```python
from build123d import *

# Parameters (mm, degrees)
CROQUIS3_R              = 2.5103265
CROQUIS3_R_2            = 2.5
SALIENTE_EXTRUIR1_DEPTH = 4


with BuildPart() as part:
    # Croquis3 → Saliente-Extruir1 (new body)
    with BuildSketch(Plane(origin=(0, 0, 0), x_dir=(0, 0, -1), z_dir=(1, 0, 0))):
        with BuildLine():
            Line((5, 0), (5, -25))
            Line((5, -25), (-20, -25))
            ThreePointArc((-20, -25), (-24.631788644, -18.116775648), (-16.510921132, -16.418613585))
            ThreePointArc((-16.510921132, -16.418613585), (-9.814593541, -8.868938988), (-5, 0))
            ThreePointArc((-5, 0), (0, 5), (5, 0))
        make_face()
        Circle(CROQUIS3_R, mode=Mode.SUBTRACT)
        with Locations((-20, -20)):
            Circle(CROQUIS3_R_2, mode=Mode.SUBTRACT)
    extrude(amount=SALIENTE_EXTRUIR1_DEPTH)


solid = part.part
```
The listing builds one solid part. Answer for the finished solid, in the listing's coordinates (mm). Round coordinates to 2 decimals unless told otherwise and drop trailing zeros. Loops run counter-clockwise (first coordinate to the right, second up) from the corner with the lowest first, then second, coordinate; pieces in that order, holes last.
1) A cutting plane is placed at D-D on z = 23. Determine the outline of the cut face in (x, y).
Outcome:
outline: (0, -24) - (4, -24) - (4, -16) - (0, -16) - close
2) For a pull along Z with two mould halves and no side action, classify faces 1 (the face through (2, -12, -5)), 2 (the face through (4, -13, 6)), 3 (the face through (2, -19.9, 22.5)) as released by +Z, released by -Z, zero draft, split by the parting line, or undercut.
Outcome:
face 1: released by -Z
face 2: zero draft
face 3: undercut
3) A cutting plane is placed at B-B on z = 0. Determine the outline of the cut face in (x, y), plus the area to 3 significant figures.
Outcome:
outline: (0, -25) - (4, -25) - (4, -2.51) - (0, -2.51) - close; (0, 2.51) - (4, 2.51) - (4, 5) - (0, 5) - close
area: 99.9 mm2
4) Consider line 1 (Y direction, x = 2.1, z = 0); line 2 (Y direction, x = 1.4, z = 20); line 3 (Z direction, x = 0.2, y = -1.5). Determine where each line is inside the solid, lowest interval first.
Outcome:
line 1: y = -25 to -2.51, 2.51 to 5
line 2: y = -25 to -22.5, -17.5 to -15
line 3: z = -5 to -2.01, 2.01 to 5.64
5) A cutting plane is placed at A-A on y = -20. Determine the outline of the cut face in (x, z).
Outcome:
outline: (0, -5) - (4, -5) - (4, 17.5) - (0, 17.5) - close; (0, 22.5) - (4, 22.5) - (4, 25) - (0, 25) - close
6) A cutting plane is placed at C-C on x = 2.95. Determine the outline of the cut face in (y, z).
Outcome:
outline: (-25, -5) - (0, -5) arc R5 ccw to (0, 5) arc R44.31 cw to (-16.42, 16.51) arc R5 ccw (long way) to (-25, 20) - close; hole circle Ø5 at (-20, 20); hole circle Ø5.02 at (0, 0)
7) Given P1, Ø6, axis at y = -11.5, z = 16.5, coming from the +X side, flat-ended and moving along its own axis, determine where the tip first touches the part or whether it passes through.
Outcome:
P1: passes through
